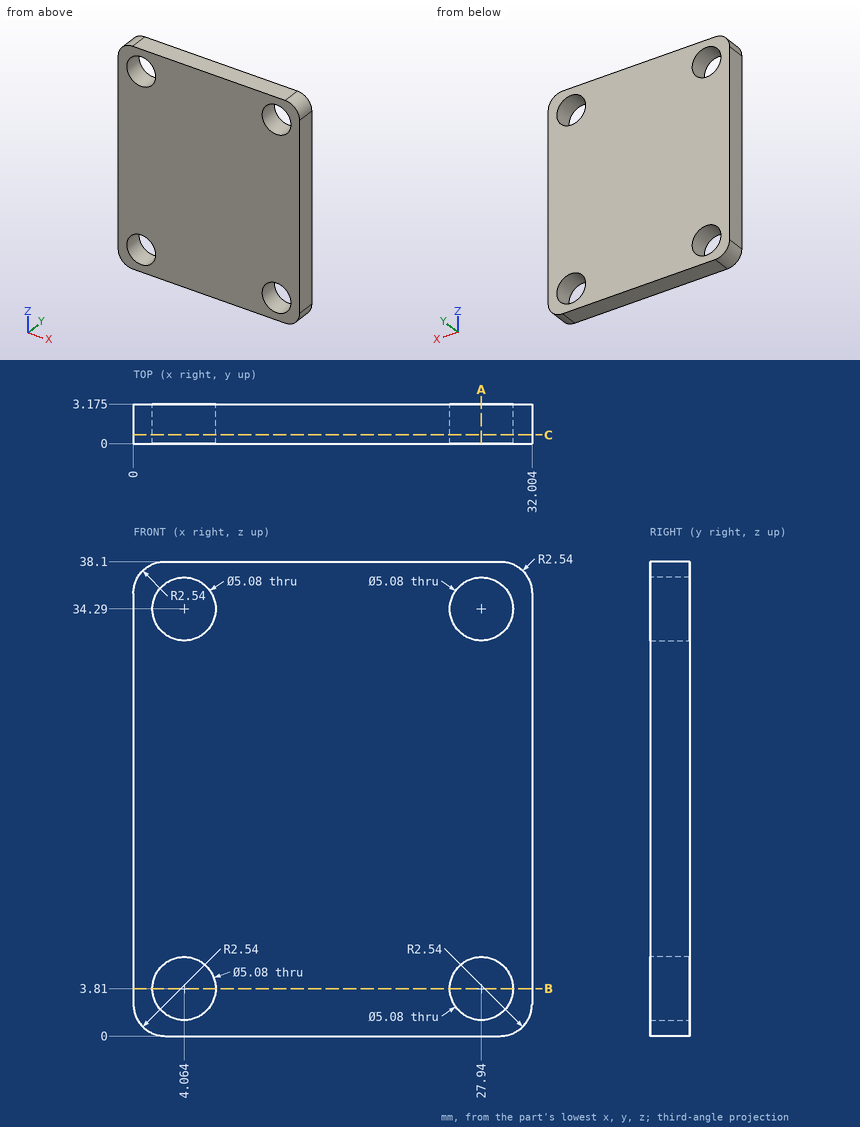
Verification items for this drawing (mm, ordinates from the low corner). Coordinates: 2 decimals unless noted, no trailing zeros. Loops run counter-clockwise (first coordinate to the right, second up) from the corner with the lowest first, then second, coordinate; pieces in that order, holes last. Notation, with made-up numbers: (73, 71) - (109, 71) arc R23 cw to (109, 99) - close; hole circle Ø1 at (42, 70.25). An arc over 180 degrees is marked (long way). Answer as a JSON object with one key per item and string values.
(1) Cross-section at B-B, the plane z = 3.81. Record the boundary of the cut face in (x, y) (3 decimals).
Response:
{"outline": "(0, 0) - (1.524, 0) - (1.524, 3.175) - (0, 3.175) - close; (6.604, 0) - (25.4, 0) - (25.4, 3.175) - (6.604, 3.175) - close; (30.48, 0) - (32.004, 0) - (32.004, 3.175) - (30.48, 3.175) - close"}
(2) Scan lines: line 1 along Z through (x, y) = (28, 0.95); line 2 along X through (y, z) = (0.85, 3.81); line 3 along Z through (x, y) = (6, 0.25). Record each from-to range of solid material in increasing order.
Response:
{"line 1": "z = 0 to 1.27, 6.35 to 31.75, 36.83 to 38.1", "line 2": "x = 0 to 1.52, 6.6 to 25.4, 30.48 to 32", "line 3": "z = 0 to 2.17, 5.45 to 32.65, 35.93 to 38.1"}
(3) Cross-section at A-A, the plane x = 27.94. Record the boundary of the cut face in (y, z) (3 decimals), then the cut area to 3 significant figures.
Response:
{"outline": "(0, 0) - (3.175, 0) - (3.175, 1.27) - (0, 1.27) - close; (0, 6.35) - (3.175, 6.35) - (3.175, 31.75) - (0, 31.75) - close; (0, 36.83) - (3.175, 36.83) - (3.175, 38.1) - (0, 38.1) - close", "area": "88.7 mm²"}
(4) Cross-section at C-C, the plane y = 0.7. Record the boundary of the cut face in (x, z), then the cut area to 3 significant figures.
Response:
{"outline": "(0, 2.54) arc R2.54 ccw to (2.54, 0) - (29.46, 0) arc R2.54 ccw to (32, 2.54) - (32, 35.56) arc R2.54 ccw to (29.46, 38.1) - (2.54, 38.1) arc R2.54 ccw to (0, 35.56) - close; hole circle Ø5.08 at (4.06, 3.81); hole circle Ø5.08 at (4.06, 34.29); hole circle Ø5.08 at (27.94, 3.81); hole circle Ø5.08 at (27.94, 34.29)", "area": "1,130 mm²"}
